Verification items for the finished model (mm, model axes). Round coordinates to 2 decimals unless told otherwise and drop trailing zeros. Write each loop counter-clockwise with the first axis right and the second up, starting at its lowest first coordinate (ties: lowest second). Pieces come first, ordered by that corner, then holes. Notation, with made-up numbers: M 38,39.5 L 92,39.5 A30 cw 92,66.5 Z; hole C 76,-8 d11. An arc over 180 degrees is marked long. One line per item, written item: value. Start each with the question number.
Item 1: Section check D-D, the plane x = 3.5. Record the cut outline in (y, z), then the cut area to 3 significant figures.
Item 2: Section check A-A, the plane y = 5.75. State how many separate pieces and enclosed holes the cut face has, then the cut area to 3 significant figures.
Item 3: Section check C-C, the plane x = 2.5. Record the cut outline in (y, z) (3 decimals), then the cut area to 3 significant figures.
Item 4: Gauge pin test, flat end, axial feed: pin 1 (0.5 mm diameter, centred on x = 0, z = 1, fed in from -Y). Record the tip position at first contact, or that the pin passes through.
Item 5: Thickness scan on probe 1 along Z at (x, y) = (-2.5, 2.5) (3 decimals); probe 2 along X at (y, z) = (3.25, -1.55) (3 decimals); probe 3 along Y at (x, z) = (-2.25, -1.25). Record the ranges inside material, lowest first. Write a range as from..to.
Item 6: Section check B-B, the plane z = -1.45. Record the cut outline in (x, y) (3 decimals).
from build123d import *

# Parameters (mm, degrees)
F0_W     = 7.68
F0_H     = 5.12
F0_W_2   = 0.65
F0_H_2   = 0.65
F1_DEPTH = 7.96
F2_DEPTH = 7
F3_SIZE  = 0.5


with BuildPart() as f1:
    # F0 (on Front) → F1 (new body)
    with BuildSketch(Plane.XZ):
        Rectangle(F0_W, F0_H)
        with Locations((-2.54, -1.27)):
            Rectangle(F0_W_2, F0_H_2, mode=Mode.SUBTRACT)
        with Locations((0, -1.27)):
            Rectangle(F0_W_2, F0_H_2, mode=Mode.SUBTRACT)
        with Locations((2.54, -1.27)):
            Rectangle(F0_W_2, F0_H_2, mode=Mode.SUBTRACT)
        with Locations((-2.54, 1.27)):
            Rectangle(F0_W_2, F0_H_2, mode=Mode.SUBTRACT)
        with Locations((0, 1.27)):
            Rectangle(F0_W_2, F0_H_2, mode=Mode.SUBTRACT)
        with Locations((2.54, 1.27)):
            Rectangle(F0_W_2, F0_H_2, mode=Mode.SUBTRACT)
        with Locations((-2.54, 1.27)):
            Rectangle(F0_W_2, F0_H_2)
        with Locations((0, 1.27)):
            Rectangle(F0_W_2, F0_H_2)
        with Locations((2.54, 1.27)):
            Rectangle(F0_W_2, F0_H_2)
        with Locations((2.54, -1.27)):
            Rectangle(F0_W_2, F0_H_2)
        with Locations((0, -1.27)):
            Rectangle(F0_W_2, F0_H_2)
        with Locations((-2.54, -1.27)):
            Rectangle(F0_W_2, F0_H_2)
    extrude(amount=-F1_DEPTH)

    # F0 (on Front) → F2 (cut)
    with BuildSketch(Plane.XZ):
        with Locations((-2.54, 1.27)):
            Rectangle(F0_W_2, F0_H_2)
        with Locations((0, 1.27)):
            Rectangle(F0_W_2, F0_H_2)
        with Locations((2.54, 1.27)):
            Rectangle(F0_W_2, F0_H_2)
        with Locations((2.54, -1.27)):
            Rectangle(F0_W_2, F0_H_2)
        with Locations((0, -1.27)):
            Rectangle(F0_W_2, F0_H_2)
        with Locations((-2.54, -1.27)):
            Rectangle(F0_W_2, F0_H_2)
    extrude(amount=-F2_DEPTH, mode=Mode.SUBTRACT)

    # F3
    f3_edges = [f1.edges().sort_by_distance(p)[0] for p in [
        (3.84, 3.98, 2.56),
        (-3.84, 3.98, 2.56),
        (3.84, 3.98, -2.56),
        (-3.84, 3.98, -2.56),
    ]]
    chamfer(f3_edges, length=F3_SIZE)


solid = f1.part
Response values:
1. outline: M 0,-2.4 L 7.96,-2.4 L 7.96,2.4 L 0,2.4 Z
1. area: 38.2 mm2
2. separate pieces: 1
2. enclosed holes: 6
2. area: 36.3 mm2
3. outline: M 0,-2.56 L 7.96,-2.56 L 7.96,2.56 L 0,2.56 L 0,1.595 L 7,1.595 L 7,0.945 L 0,0.945 L 0,-0.945 L 7,-0.945 L 7,-1.595 L 0,-1.595 Z
3. area: 31.7 mm2
4. pin 1: stops at y = 0
5. probe 1: z = -2.56..-1.595, -0.945..0.945, 1.595..2.56
5. probe 2: x = -3.84..-2.865, -2.215..-0.325, 0.325..2.215, 2.865..3.84
5. probe 3: y = 7..7.96
6. outline: M -3.84,0 L -2.865,0 L -2.865,7 L -2.215,7 L -2.215,0 L -0.325,0 L -0.325,7 L 0.325,7 L 0.325,0 L 2.215,0 L 2.215,7 L 2.865,7 L 2.865,0 L 3.84,0 L 3.84,7.96 L -3.84,7.96 Z
